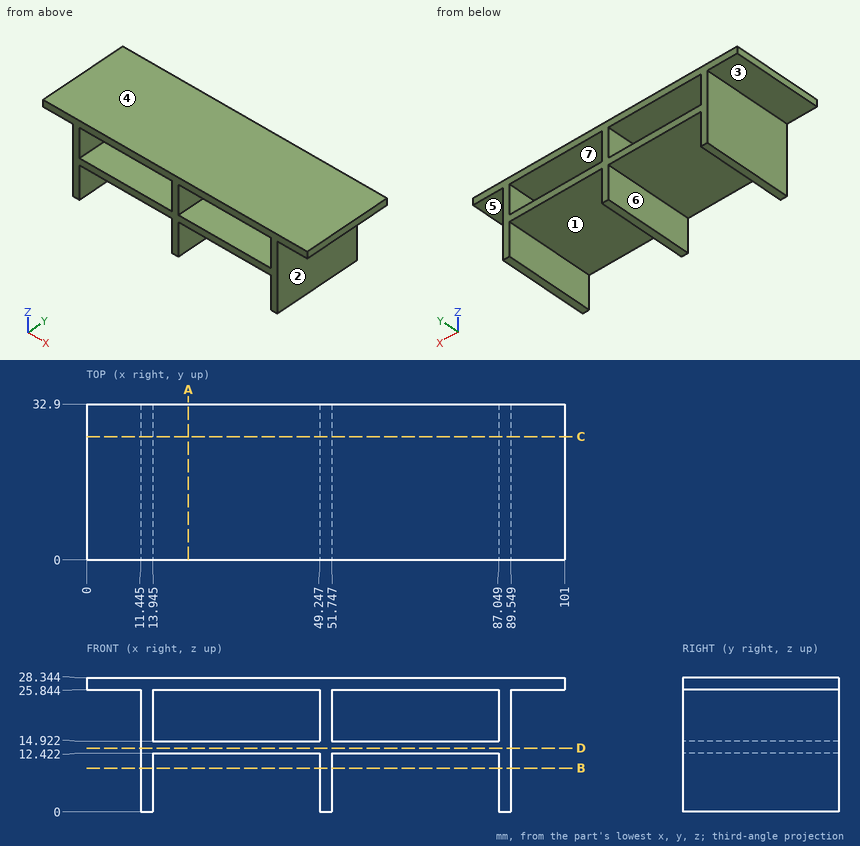
Drawing for the job (mm, zero at the part's lowest x, y, z). A direction names the side the tool comes from. Give positions to 0.01 mm unless a question says otherwise; leave off trailing zeros. Write each loop counter-clockwise with the first axis right and the second up, starting at its lowest first coordinate (ties: lowest second). Pieces come first, ordered by that corner, then holes. Notation, with made-up numbers: (18.25, 50) -> (53.25, 50) arc R18 cw to (53.25, 76) -> close; hole circle Ø5 at (-19.75, -1). An arc over 180 degrees is marked (long way). Put each result on its own line as item: value. Start each with the question number.
Item 1: Cut at A-A (x = 21.5). List the corners of the cut face in (y, z).
Item 2: Cut at D-D (z = 13.5). List the corners of the cut face in (x, y) (3 decimals), then the cut area to 3 significant figures.
Item 3: Cut at B-B (z = 9.25). List the corners of the cut face in (x, y) (3 decimals), then the cut area to 3 significant figures.
Item 4: Which spindle directions (+Z, -Z, +X, -X, +Y, -Y) get a long thin tool onto all of the face, cutting with end or side? Do the marked faces 4, 5, 6 and 7. Say none if no direction does.
Item 5: Wall check: L1, parallel to X at y = 26, z = 11.25 (3 decimals); L2, parallel to Z at x = 45, y = 4; L3, parallel to X at y = 27, z = 14.75 (3 decimals). Give the ranges that are in metal, low to high. Write a range as [from, to].
Item 6: Pin check, flat tips, straight feed: pin 1 Ø10 at (x, y) = (26.5, 17.5) entering from -Z; pin 2 Ø13.5 at (y, z) = (18, 7.5) entering from -X (3 decimals); pin 3 Ø12.5 at (x, y) = (97, 21) entering from -Z; pin 4 Ø1.5 at (x, z) = (24, 24) entering from -Y. Stop position of each tip, or through.
Item 7: Pull direction X, two halves, no side cores. Call the marked faces 1, 2 and 3: pulls with the +X half, pulls with the -X half, needs draft (parallel to the pull), parting line crosses it, or undercut.
Item 8: Cut at C-C (y = 26). List the corners of the cut face in (x, z) (3 decimals).
Answer list:
1. outline: (0, 12.42) -> (32.9, 12.42) -> (32.9, 14.92) -> (0, 14.92) -> close; (0, 25.84) -> (32.9, 25.84) -> (32.9, 28.34) -> (0, 28.34) -> close
2. outline: (11.445, 0) -> (89.549, 0) -> (89.549, 32.9) -> (11.445, 32.9) -> close
2. area: 2,570 mm2
3. outline: (11.445, 0) -> (13.945, 0) -> (13.945, 32.9) -> (11.445, 32.9) -> close; (49.247, 0) -> (51.747, 0) -> (51.747, 32.9) -> (49.247, 32.9) -> close; (87.049, 0) -> (89.549, 0) -> (89.549, 32.9) -> (87.049, 32.9) -> close
3. area: 247 mm2
4. face 4: +Z, +X, -X, +Y, -Y
4. face 5: -Z, +X, +Y, -Y
4. face 6: -Z, +Y, -Y
4. face 7: +Y, -Y
5. L1: x = [11.445, 13.945], [49.247, 51.747], [87.049, 89.549]
5. L2: z = [12.42, 14.92], [25.84, 28.34]
5. L3: x = [11.445, 89.549]
6. pin 1: stops at z = 12.42
6. pin 2: stops at x = 11.445
6. pin 3: stops at z = 25.84
6. pin 4: passes through
7. face 1: undercut
7. face 2: pulls with the +X half
7. face 3: needs draft
8. outline: (0, 25.844) -> (11.445, 25.844) -> (11.445, 0) -> (13.945, 0) -> (13.945, 12.422) -> (49.247, 12.422) -> (49.247, 0) -> (51.747, 0) -> (51.747, 12.422) -> (87.049, 12.422) -> (87.049, 0) -> (89.549, 0) -> (89.549, 25.844) -> (101, 25.844) -> (101, 28.344) -> (0, 28.344) -> close; hole (13.945, 14.922) -> (49.247, 14.922) -> (49.247, 25.844) -> (13.945, 25.844) -> close; hole (51.747, 14.922) -> (87.049, 14.922) -> (87.049, 25.844) -> (51.747, 25.844) -> close
